```python
from build123d import *

# Parameters (mm, degrees)
EXTRUDE_1_DEPTH          = 7
EXTRUDE_1_DEPTH_BACK     = 7
SKETCH_1_R               = 1.5
FILLET_1_R               = 10
EXTRUDE_2_DEPTH          = 2.9
EXTRUDE_2_DEPTH_BACK     = 2.8
SKETCH_3_R               = 1.5
CUT_EXTRUDE_1_DEPTH      = 5.2
CUT_EXTRUDE_1_DEPTH_BACK = 5.2


with BuildPart() as part:
    # Sketch 1 → Extrude 1 (new, two sides: drawn at the far end of the back side and taken through both)
    with BuildSketch(Plane.XY.offset(-EXTRUDE_1_DEPTH_BACK)):
        with BuildLine():
            ThreePointArc((240.699236038, 105.645995337), (243.6, 101.8), (240.699236038, 97.954004663))
            Line((240.699236038, 97.954004663), (232.071936087, 95.488208898))
            Line((232.071936087, 95.488208898), (163.6, 91.5))
            ThreePointArc((163.6, 91.5), (147.125308547, 88.283437456), (132.1, 80.8))
            Line((132.1, 80.8), (97.347754748, 57.19128445))
            ThreePointArc((97.347754748, 57.19128445), (92.03920173, 57.924827394), (92.224555949, 63.280615311))
            Line((92.224555949, 63.280615311), (128.7, 101))
            ThreePointArc((128.7, 101), (143.303490983, 110.55954938), (160.6, 112.9))
            Line((160.6, 112.9), (232.071936087, 108.111791102))
            Line((232.071936087, 108.111791102), (240.699236038, 105.645995337))
        make_face()
        with Locations((95.1, 60.5)):
            Circle(SKETCH_1_R, mode=Mode.SUBTRACT)
        with Locations((152.6, 99.603139307)):
            Circle(SKETCH_1_R, mode=Mode.SUBTRACT)
        with Locations((239.6, 101.8)):
            Circle(SKETCH_1_R, mode=Mode.SUBTRACT)
    extrude(amount=EXTRUDE_1_DEPTH + EXTRUDE_1_DEPTH_BACK)

    # Fillet 1
    fillet_1_edges = [part.edges().sort_by_distance(p)[0] for p in [
        (232.071936087, 95.488208898, 0),
        (232.071936087, 108.111791102, 0),
    ]]
    fillet(fillet_1_edges, radius=FILLET_1_R)

    # Sketch 3 → Extrude 2 (add, two sides: drawn at the far end of the back side and taken through both)
    with BuildSketch(Plane.XY.offset(-EXTRUDE_2_DEPTH_BACK)):
        with BuildLine():
            Line((160.6, 112.9), (163.651401787, 112.69557362))
            Line((163.651401787, 112.69557362), (163.893737551, 116.312835642))
            ThreePointArc((163.893737551, 116.312835642), (162.654460758, 118.828873494), (159.855517856, 119.008239262))
            Line((159.855517856, 119.008239262), (139.549521827, 108.933263618))
            ThreePointArc((139.549521827, 108.933263618), (149.801009446, 112.369362402), (160.6, 112.9))
        make_face()
        with Locations((161.1, 116.5)):
            Circle(SKETCH_3_R, mode=Mode.SUBTRACT)
    extrude(amount=EXTRUDE_2_DEPTH + EXTRUDE_2_DEPTH_BACK)

    # Sketch 4 → Cut-Extrude 1 (cut, two sides: drawn at the far end of the back side and taken through both)
    with BuildSketch(Plane.XY.offset(-CUT_EXTRUDE_1_DEPTH_BACK)):
        with BuildLine():
            Line((231.012866709, 108.182742662), (224.6, 108.612367871))
            Line((224.6, 108.612367871), (228.236474469, 103.550312019))
            ThreePointArc((228.236474469, 103.550312019), (228.799985675, 101.790729145), (228.225610058, 100.034662683))
            Line((228.225610058, 100.034662683), (224.6, 95.052999327))
            Line((224.6, 95.052999327), (230.968280992, 95.423925524))
            ThreePointArc((230.968280992, 95.423925524), (232.061731819, 95.548272011), (233.134897693, 95.792017302))
            Line((233.134897693, 95.792017302), (240.699236038, 97.954004663))
            ThreePointArc((240.699236038, 97.954004663), (243.6, 101.8), (240.699236038, 105.645995337))
            Line((240.699236038, 105.645995337), (233.092512669, 107.820096895))
            ThreePointArc((233.092512669, 107.820096895), (232.062285935, 108.056450871), (231.012866709, 108.182742662))
        make_face()
    extrude(amount=CUT_EXTRUDE_1_DEPTH + CUT_EXTRUDE_1_DEPTH_BACK, mode=Mode.SUBTRACT)


solid = part.part
```
Input: part model. Units: mm. Frame: model coordinates. A direction names the side the tool comes from. Round coordinates to 2 decimals unless told otherwise and drop trailing zeros. Loops run counter-clockwise (first coordinate to the right, second up) from the corner with the lowest first, then second, coordinate; pieces in that order, holes last. Notation, with made-up numbers: (88.5, -1.5) -> (112.5, -1.5) arc R14 cw to (112.5, 24.5) -> close; hole circle Ø4 at (62, 51). An arc over 180 degrees is marked (long way). Write each question's results on one line, items separated by ' | '.
1. Section C-C (x = 95.1). Return loops of the section in (y, z), and give its area (3 significant figures).
Geometry results:
outline: (56.5, -7) -> (59, -7) -> (59, 7) -> (56.5, 7) -> close; (62, -7) -> (66.25, -7) -> (66.25, 7) -> (62, 7) -> close | area: 94.6 mm2
2. Section B-B (x = 152.6). Return loops of the section in (y, z), and give its area (3 significant figures).
Geometry results:
outline: (89.87, -7) -> (98.1, -7) -> (98.1, 7) -> (89.87, 7) -> close; (101.1, -7) -> (112.79, -7) -> (112.79, -2.8) -> (115.41, -2.8) -> (115.41, 2.9) -> (112.79, 2.9) -> (112.79, 7) -> (101.1, 7) -> close | area: 294 mm2
3. Section D-D (x = 113.5). Return loops of the section in (y, z).
Geometry results:
outline: (68.16, -7) -> (85.28, -7) -> (85.28, 7) -> (68.16, 7) -> close
4. Section A-A (y = 60.5). Return loops of the section in (x, z), and give its area (3 significant figures).
Geometry results:
outline: (91.1, -7) -> (93.6, -7) -> (93.6, 7) -> (91.1, 7) -> close; (96.6, -7) -> (102.22, -7) -> (102.22, 7) -> (96.6, 7) -> close | area: 114 mm2
5. First-contact query: P1, Ø8, axis at y = 81, z = -2.5, coming from the -X side; P2, Ø4, axis at y = 83.5, z = 2.5, coming from the +X side; P3, Ø4, axis at x = 239.6, y = 101.8, coming from the +Z side; P4, Ø1.5, axis at x = 107.5, z = 0, coming from the -Y side. Flat tips, straight axial feed; report the tip coordinate or a pass-through.
Geometry results:
P1: x = 105.49 | P2: x = 140.29 | P3: z = 7 | P4: y = 63.58
6. Mould query, pull axis Z, two halves, no side actions, for faces 6 (the face through (234, 102, -5.2)), 7 (the face through (149.84, 114.04, 0.01)), 8 (the face through (157, 115, -2.8)). Classes: +Z half, -Z half, draft (parallel to the pull), parting line (faces both ways), or undercut.
Geometry results:
face 6: undercut | face 7: draft | face 8: -Z half
7. Set-up query: faces 1 (the face through (228.8, 101.8, -0.1)), 2 (the face through (197.76, 93.49, -0.1)), 3 (the face through (226.44, 97.58, -0.07)), 4 (the face through (226.39, 106.12, -0.07)), 5 (the face through (152.4, 101.09, -0.1)). Return all of +Z, -Z, +X, -X, +Y, -Y with unobstructed straight access to the full face (end or side cutting, diameter ignored); none if empty.
Geometry results:
face 1: +X | face 2: +Z, -Z, +X, -Y | face 3: +X, -Y | face 4: +X, +Y | face 5: +Z, -Z
8. Ray query, line 1 (X direction, y = 116.5, z = -1.1); line 2 (Y direction, x = 239.6, z = -6); line 3 (Y direction, x = 152.6, z = -3.5). Return the intervals inside material, ascending. Write a range as from..to.
Geometry results:
line 1: 154.8..159.6, 162.6..163.9 | line 2: 97.64..100.3, 103.3..105.96 | line 3: 89.87..98.1, 101.1..112.79
